Read the model definition and answer for the solid it produces. Units are mm, in the model's axes. Face numbers are marked on the shaded views. A direction names the side the tool comes from. Give positions to 0.01 mm unless a question says otherwise; leave off trailing zeros. Order: outer loops, then holes, each group sorted by start corner. A loop starts at its lowest first (then second) coordinate and runs counter-clockwise, first axis right, second up. Notation, with made-up numbers: (-9, -10.75) - (27, -10.75) arc R21 cw to (27, 18.25) - close; hole circle Ø4 at (23, -13). An arc over 180 degrees is marked (long way). Use a Markdown table: item, result. Add a question column.
1. A cutting plane is placed at D-D on x = -14. Determine the outline of the cut face in (y, z).
2. Consider L1, parallel to X at y = -2.4, z = 0; L2, parallel to Y at x = 15, z = 3.75; L3, parallel to Y at x = 7, z = -0.75. Determine where each line is inside the solid, lowest interval first.
3. A cutting plane is placed at C-C on y = 9.25. Determine the outline of the cut face in (x, z).
4. Flat-ended cylindrical pins translate along their axes: P1, Ø4, axis at y = 3, z = 1, coming from the -X side; P2, Ø4, axis at y = 11, z = -2, coming from the -X side; P3, Ø4, axis at y = 12.5, z = 1.5, coming from the +X side; P4, Ø5, axis at x = 14.5, z = 1.5, coming from the +Y side. Find the tip coordinate at first contact, or state that the pin passes through.
5. For a pull along X with two mould halves and no side action, classify the marked faces 1, 2 and 3 as released by +X, released by -X, zero draft, split by the parting line, or undercut.
6. A cutting plane is placed at B-B on x = -1.7. Determine the outline of the cut face in (y, z).
7. Which of the six approach directions +Z, -Z, +X, -X, +Y, -Y give full straight-line access (tool end or side, diameter ignored) to the marked faces 4, 5, 6, 7 and 8?
8. A cutting plane is placed at A-A on z = -5. Determine the outline of the cut face in (x, y).
```python
from build123d import *

# Parameters (mm, degrees)
SKETCH1_W           = 22.4
SKETCH1_H           = 12.5
BOSS_EXTRUDE1_DEPTH = 22.8
SKETCH2_W           = 12.5
SKETCH2_H           = 2
BOSS_EXTRUDE2_DEPTH = 4.7
SKETCH3_W           = 12.5
SKETCH3_H           = 2
BOSS_EXTRUDE3_DEPTH = 4.7
BOSS_EXTRUDE5_DEPTH = 3.5
SKETCH5_R           = 2.5
CUT_EXTRUDE1_DEPTH  = 5


with BuildPart() as part:
    # Sketch1 → Boss-Extrude1 (new body)
    with BuildSketch(Plane(origin=(0, 0, 0), x_dir=(1, 0, 0), z_dir=(0, 1, 0))):
        Rectangle(SKETCH1_W, SKETCH1_H)
    extrude(amount=BOSS_EXTRUDE1_DEPTH)

    # Sketch2 → Boss-Extrude2 (add)
    with BuildSketch(Plane(origin=(11.2, 0, 0), x_dir=(0, 0, -1), z_dir=(1, 0, 0))):
        with Locations((0, 5.7)):
            Rectangle(SKETCH2_W, SKETCH2_H)
    extrude(amount=BOSS_EXTRUDE2_DEPTH)

    # Sketch3 → Boss-Extrude3 (add)
    with BuildSketch(Plane.ZY.offset(11.2)):
        with Locations((0, 5.7)):
            Rectangle(SKETCH3_W, SKETCH3_H)
    extrude(amount=BOSS_EXTRUDE3_DEPTH)

    # Sketch4 → Boss-Extrude5 (add)
    with BuildSketch(Plane.XZ):
        with BuildLine():
            ThreePointArc((-0.842105263, -2.348194332), (11.2, 0), (-0.842105263, 2.348194332))
            ThreePointArc((-0.842105263, 2.348194332), (-4.2, 0), (-0.842105263, -2.348194332))
        make_face()
    extrude(amount=BOSS_EXTRUDE5_DEPTH)

    # Sketch5 → Cut-Extrude1 (cut)
    with BuildSketch(Plane.XZ.offset(3.5)):
        with Locations(Location((4.95, 0, 0), (0, 0, 270))):
            Circle(SKETCH5_R)
    extrude(amount=-CUT_EXTRUDE1_DEPTH, mode=Mode.SUBTRACT)


solid = part.part
```
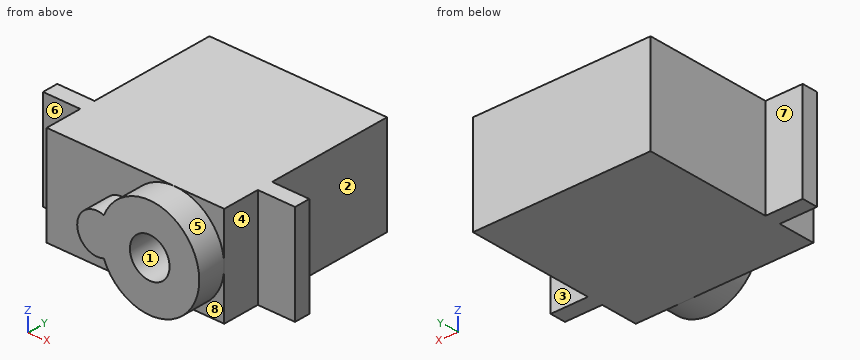
Output values:
| question | item | result |
|---|---|---|
| 1 | outline | (4.7, -6.25) - (6.7, -6.25) - (6.7, 6.25) - (4.7, 6.25) - close |
| 2 | L1 | -4.2 to 2.45, 7.45 to 11.2 |
| 2 | L2 | 4.7 to 6.7 |
| 2 | L3 | 1.5 to 22.8 |
| 3 | outline | (-11.2, -6.25) - (11.2, -6.25) - (11.2, 6.25) - (-11.2, 6.25) - close |
| 4 | P1 | x = -15.9 |
| 4 | P2 | x = -11.2 |
| 4 | P3 | x = 11.2 |
| 4 | P4 | y = 6.7 |
| 5 | face 1 | undercut |
| 5 | face 2 | released by +X |
| 5 | face 3 | zero draft |
| 6 | outline | (-3.5, -2.5) - (0, -2.5) - (0, -6.25) - (22.8, -6.25) - (22.8, 6.25) - (0, 6.25) - (0, 2.5) - (-3.5, 2.5) - close |
| 7 | face 4 | +Z, -Z, +X, -Y |
| 7 | face 5 | -Y |
| 7 | face 6 | +Z, -Z, -X, -Y |
| 7 | face 7 | +Z, -Z, -X, +Y |
| 7 | face 8 | -Z, +X, -Y |
| 8 | outline | (-15.9, 4.7) - (-11.2, 4.7) - (-11.2, 0) - (1.2, 0) - (1.2, -3.5) - (8.7, -3.5) - (8.7, 0) - (11.2, 0) - (11.2, 4.7) - (15.9, 4.7) - (15.9, 6.7) - (11.2, 6.7) - (11.2, 22.8) - (-11.2, 22.8) - (-11.2, 6.7) - (-15.9, 6.7) - close |
